from build123d import *

# Parameters (mm, degrees)
F0_W     = 22.225
F0_H     = 22.225
F1_DEPTH = 6.35


with BuildPart() as f1:
    # F0 (on Front) → F1 (new body)
    with BuildSketch(Plane.XZ):
        Rectangle(F0_W, F0_H)
        Polygon((-7.332348, 0), (-3.666174, 6.35), (3.666174, 6.35), (7.332348, 0), (3.666174, -6.35), (-3.666174, -6.35), align=None, mode=Mode.SUBTRACT)
    extrude(amount=F1_DEPTH)


solid = f1.part
Read the model definition and answer for the solid it produces. Units are mm, in the model's axes. A direction names the side the tool comes from. Round coordinates to 2 decimals unless told otherwise and drop trailing zeros. Loops run counter-clockwise (first coordinate to the right, second up) from the corner with the lowest first, then second, coordinate; pieces in that order, holes last.
Q1. Which of the six approach directions +Z, -Z, +X, -X, +Y, -Y give full straight-line access (tool end or side, diameter ignored) to faces 1 (the face through (-11.112, -3, 0)), 2 (the face through (-5.525, -3.131, 3.131))?
Q2. Determine the mould class of faces 3 (the face through (5.474, -3.131, 3.219)), 4 (the face through (0, -3, -11.112)), 5 (the face through (11.112, -3, 0)), 6 (the face through (-5.474, -3.131, -3.219)) for opening direction Z: released by +Z, released by -Z, zero draft, split by the parting line, or undercut.
Q3. Section C-C on z = -3.75 is taken. Write down the section's boundary in (x, y), and give its area (3 significant figures).
Q4. Section A-A on x = 1.25 is taken. Write down the section's boundary in (y, z).
Q5. Section B-B on y = -1 is taken. Write down the section's boundary in (x, z).
Q6. Consider probe 1 along Z at (x, y) = (-3, -3); probe 2 along Z at (x, y) = (-5.25, -2); probe 3 along X at (y, z) = (-4, -1) (1 decimal). Determine where each line is inside the solid, lowest interval first.
Output:
1. face 1: +Z, -Z, -X, +Y, -Y
1. face 2: +Y, -Y
2. face 3: undercut
2. face 4: released by -Z
2. face 5: zero draft
2. face 6: undercut
3. outline: (-11.11, -6.35) - (-5.17, -6.35) - (-5.17, 0) - (-11.11, 0) - close; (5.17, -6.35) - (11.11, -6.35) - (11.11, 0) - (5.17, 0) - close
3. area: 75.5 mm2
4. outline: (-6.35, -11.11) - (0, -11.11) - (0, -6.35) - (-6.35, -6.35) - close; (-6.35, 6.35) - (0, 6.35) - (0, 11.11) - (-6.35, 11.11) - close
5. outline: (-11.11, -11.11) - (11.11, -11.11) - (11.11, 11.11) - (-11.11, 11.11) - close; hole (-7.33, 0) - (-3.67, -6.35) - (3.67, -6.35) - (7.33, 0) - (3.67, 6.35) - (-3.67, 6.35) - close
6. probe 1: z = -11.11 to -6.35, 6.35 to 11.11
6. probe 2: z = -11.11 to -3.61, 3.61 to 11.11
6. probe 3: x = -11.1 to -6.8, 6.8 to 11.1
